from build123d import *

# Parameters (mm, degrees)
SKETCH1_R                = 1.5875
BOSS_EXTRUDE1_DEPTH      = 3.175
BOSS_EXTRUDE1_DEPTH_BACK = 3.175
FILLET1_R                = 0.79375


with BuildPart() as part:
    # Sketch1 → Boss-Extrude1 (new body, two sides)
    with BuildSketch(Plane.XY) as boss_extrude1_sk:
        with BuildLine():
            Line((-7.728108964, 8.128), (-6.707222541, 11.938))
            Line((-6.707222541, 11.938), (-27.145240318, 6.858))
            ThreePointArc((-27.145240318, 6.858), (-28.349785751, 5.325893193), (-27.161747679, 3.780950957))
            Line((-27.161747679, 3.780950957), (-1.215078314, -2.964648418))
            Line((-1.215078314, -2.964648418), (41.117892306, -27.405600401))
            Line((41.117892306, -27.405600401), (44.292892306, -21.906339087))
            Line((44.292892306, -21.906339087), (-7.728108964, 8.128))
        make_face()
        Circle(SKETCH1_R, mode=Mode.SUBTRACT)
    extrude(amount=BOSS_EXTRUDE1_DEPTH)
    extrude(boss_extrude1_sk.sketch, amount=-BOSS_EXTRUDE1_DEPTH_BACK)

    # Fillet1
    fillet1_edges = [part.edges().sort_by_distance(p)[0] for p in [
        (44.292892306, -21.906339087, 0),
        (41.117892306, -27.405600401, 0),
        (-6.707222541, 11.938, 0),
        (-7.728108964, 8.128, 0),
    ]]
    fillet(fillet1_edges, radius=FILLET1_R)


solid = part.part
Check sheet for the modelled part. Datum: model origin and axes. Units: mm. Give positions to 0.01 mm unless a question says otherwise; leave off trailing zeros. Loops run counter-clockwise (first coordinate to the right, second up) from the corner with the lowest first, then second, coordinate; pieces in that order, holes last. Notation, with made-up numbers: M 58.25,64 L 68.25,64 A19 ccw 68.25,99 Z; hole C 67.25,9 d4. An arc over 180 degrees is marked long. Answer as a JSON object with one key per item and string values. Group by question number.
Q1. Material ranges on line 1 along Y through (x, z) = (0.5, -2.5); line 2 along Y through (x, z) = (0, -0.95); line 3 along X through (y, z) = (5.5, 2.5), recorded low to high. Write a range as [from, to].
Q2. Release check for a two-part mould opening along Y. For faces 1 (the flat face through (-14.37, 0.455, 0.044)), 2 (the flat face through (8, -6, 3.175)), 3 (the flat face through (-17.446, 9.269, 0.044)), 4 (the flat face through (-7.317, 9.663, 0.044)) record: released by +Y, released by -Y, zero draft, split by the parting line, or undercut.
Q3. Cross-section at A-A on z = -2.25. Record the cut outline in (x, y) (1 decimal).
Q4. Cross-section at C-C on x = 0. Record the cut outline in (y, z) (1 decimal).
Q5. Go/stop test with flat-tipped pins: P1, Ø6, axis at x = 13.5, y = -13, coming from the +Z side (3 decimals); P2, Ø2, axis at y = -20.5, z = -2.5, coming from the +X side. Record where each tip stops, or that it passes through.
Q6. Cross-section at D-D on x = -11. Record the cut outline in (y, z) (3 decimals).
Evaluation:
{
 "1": {"line 1": "y = [-3.95, -1.51], [1.51, 3.38]", "line 2": "y = [-3.67, -1.59], [1.59, 3.67]", "line 3": "x = [-28.34, -3.18]"},
 "2": {"face 1": "released by -Y", "face 2": "zero draft", "face 3": "released by +Y", "face 4": "undercut"},
 "3": {"outline": "M -27.2,3.8 L -1.2,-3 L 40.4,-27 A0.8 ccw 41.5,-26.7 L 43.9,-22.6 A0.8 ccw 43.6,-21.5 L -7.2,7.8 A0.8 cw -7.6,8.7 L -7.1,10.6 A0.8 ccw -8,11.6 L -27.1,6.9 A1.6 ccw Z; hole C 0,0 d3.2"},
 "4": {"outline": "M -3.7,-3.2 L -1.6,-3.2 L -1.6,3.2 L -3.7,3.2 Z; M 1.6,-3.2 L 3.7,-3.2 L 3.7,3.2 L 1.6,3.2 Z"},
 "5": {"P1": "stops at z = 3.175", "P2": "stops at x = 43.59"},
 "6": {"outline": "M -0.421,-3.175 L 10.871,-3.175 L 10.871,3.175 L -0.421,3.175 Z"}
}
